Build history of the part. All positions in model axes, mm. Coordinates: 2 decimals unless noted, no trailing zeros. Order: outer loops, then holes, each group sorted by start corner. A loop starts at its lowest first (then second) coordinate and runs counter-clockwise, first axis right, second up. Notation, with made-up numbers: (70.25, 87.25) - (106.25, 87.25) arc R28 cw to (106.25, 106.25) - close; hole circle Ø1 at (-25, 24). An arc over 180 degrees is marked (long way). Write each question's results on one line, items separated by ' | '. Start each with the question number.
from build123d import *

# Parameters (mm, degrees)
F2_W           = 20
F2_H           = 40
F6_D           = 4
F6_DEPTH       = 100
F6_TIP         = 1.2017212381
F6_ON_F5_D     = 4
F6_ON_F5_DEPTH = 100
F6_ON_F5_TIP   = 1.2017212381


with BuildPart() as f3:
    # F3: sweep along a path in F0
    with BuildLine(Plane.YZ) as f3_path:
        Line((-500, 80), (-500, 0))
        Line((-500, 0), (500, 0))
        Line((500, 0), (500, 80))
    # F2 (on plane+point) → F3 (sweep)
    with BuildSketch(Plane.XY.offset(80)):
        with Locations((0, -500)):
            Rectangle(F2_W, F2_H)
    sweep(path=f3_path.line, transition=Transition.RIGHT)

    # F6
    with Locations(Plane.XY.offset(80)):
        with Locations((0, -500)):
            Hole(F6_D / 2, depth=F6_DEPTH)
            with Locations((0, 0, -(F6_DEPTH + F6_TIP / 2))):  # 118° drill point
                Cone(0, F6_D / 2, F6_TIP, mode=Mode.SUBTRACT)

    # F6 on F5
    with Locations(Plane.XY.offset(80)):
        with Locations((0, 500)):
            Hole(F6_ON_F5_D / 2, depth=F6_ON_F5_DEPTH)
            with Locations((0, 0, -(F6_ON_F5_DEPTH + F6_ON_F5_TIP / 2))):  # 118° drill point
                Cone(0, F6_ON_F5_D / 2, F6_ON_F5_TIP, mode=Mode.SUBTRACT)


solid = f3.part
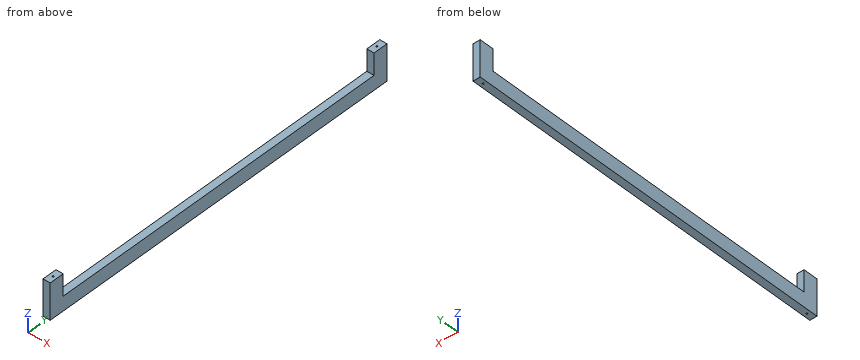
Item 1: Slice it at B-B (y = -42.5). Write the cut outline in (x, z).
Item 2: Slice it at A-A (z = 66.5). Write the cut outline in (x, y).
Item 3: Probe probe 1 along Y at (x, z) = (0, 28.5); probe 2 along Y at (x, z) = (0, 12); probe 3 along Y at (x, z) = (0.75, -13). List the from-to ranges inside material, lowest first.
Item 4: Flat gauge pin, fed straight in: P1, Ø1, axis at x = 0.5, y = -227.5, coming from the +Z side. Where does the tip first touch, or does it go through?
Resolved:
1) outline: (-10, -20) - (10, -20) - (10, 20) - (-10, 20) - close
2) outline: (-10, -520) - (10, -520) - (10, -480) - (-10, -480) - close; (-10, 480) - (10, 480) - (10, 520) - (-10, 520) - close; hole circle Ø4 at (0, -500); hole circle Ø4 at (0, 500)
3) probe 1: -520 to -502, -498 to -480, 480 to 498, 502 to 520 | probe 2: -520 to -502, -498 to 498, 502 to 520 | probe 3: -520 to -501.85, -498.15 to 498.15, 501.85 to 520
4) P1: z = 20
